Could you check a few things on this model? Use its own coordinates, in mm. Face numbers are marked on the shaded views. A direction names the side the tool comes from. Round coordinates to 2 decimals unless told otherwise and drop trailing zeros. Write each loop counter-clockwise with the first axis right and the second up, starting at its lowest first coordinate (ties: lowest second). Pieces come first, ordered by that corner, then holes. Notation, with made-up numbers: (13, 84.5) -> (25, 84.5) arc R12 ccw to (25, 96.5) -> close; hole circle Ø4 at (83.25, 45). An arc over 180 degrees is marked (long way). Answer in a Markdown table with one row per item.
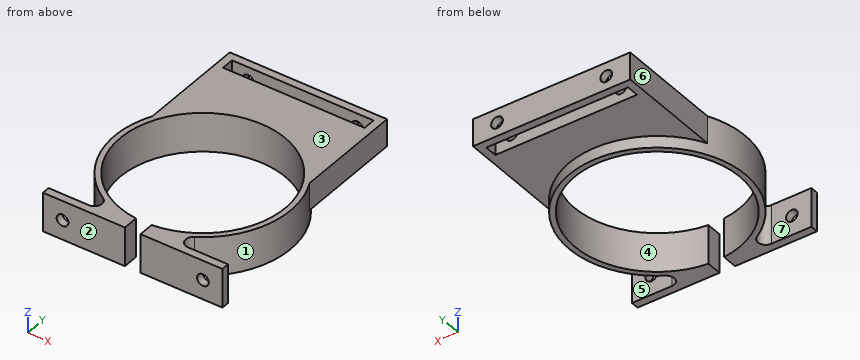
Autodesk Inventor part; units mm, degrees
ref_plane "YZ Plane" through (0, 0, 0) normal (1, 0, 0) x (0, 1, 0)
ref_plane "XZ Plane" through (0, 0, 0) normal (0, 1, 0) x (-1, 0, 0)
ref_plane "XY Plane" through (0, 0, 0) normal (0, 0, 1) x (1, 0, 0)
sketch "Sketch1" plane through (0, 0, 0) normal (0, 0, 1) x (1, 0, 0)
  circle A0 centre (0, 0) radius 21.15 construction
  line L0 (-18, -25) -> (18, -25) construction
  line L1 (-18, -25) -> (-18, -38.1522) construction
  line L2 (18, -25) -> (18, -38.1522) construction
  line L3 (-23, -23) -> (-23, -25)
  line L4 (-23, -25) -> (-2, -25)
  line L5 (-2, -21.0552) -> (-2, -25)
  line L6 (2, -21.0552) -> (2, -25)
  line L7 (2, -25) -> (23, -25)
  line L8 (23, -25) -> (23, -23)
  line L9 (23, -23) -> (12.7162, -23)
  line L10 (-23, -23) -> (-12.7162, -23)
  arc A1 (11.6803, -19.2892) -> (-11.6803, -19.2892) centre (0, 0) ccw
  arc A2 (2, -21.0552) -> (-2, -21.0552) centre (0, 0) ccw
  arc A3 (11.6803, -19.2892) -> (12.7162, -23) centre (12.7162, -21) ccw
  arc A4 (-12.7162, -23) -> (-11.6803, -19.2892) centre (-12.7162, -21) ccw
  point P0 (0, -25)
  dimension "d13" = 42.3
  dimension "d1" = 25
  dimension "d2" = 36
  dimension "d3" = 2
  dimension "d4" = 1.4
  dimension "d5" = 5
  dimension "d6" = 2
  dimension "d7" = 4
extrude "Extrusion1" add sketch "Sketch1" along normal blind 10
sketch "Sketch2" plane through (2, -25, 0) normal (0, -1, 0) x (1, 0, 0)
  circle A0 centre (16, 5) radius 1.5
  line L0 (21, 0) -> (21, 10)
  point P0 (-2, 0)
  point P1 (16, 0)
  point P2 (16, 0)
  point P3 (16, 0)
  point P4 (21, 5)
  dimension "d10" = 3
extrude "Extrusion2" cut sketch "Sketch2" against normal up to surface (2 mm away)
mirror "Mirror1" about plane through (0, 0, 0) normal (1, 0, 0) of "Extrusion2"
sketch "Sketch3" plane through (0, 0, 10) normal (0, 0, 1) x (1, 0, 0)
  arc A0 (21.9303, 5.25) -> (-21.9303, 5.25) centre (0, 0) ccw
  line L0 (-18.15, 35.75) -> (18.15, 35.75)
  line L1 (18.15, 35.75) -> (18.15, 32.55)
  line L2 (18.15, 32.55) -> (-18.15, 32.55)
  line L3 (-18.15, 32.55) -> (-18.15, 35.75)
  line L4 (-20.15, 37.75) -> (20.15, 37.75)
  line L5 (20.15, 37.75) -> (20.15, 10.1232)
  arc A1 (11.6803, -19.2892) -> (-11.6803, -19.2892) centre (0, 0) ccw
  line L6 (-20.15, 37.75) -> (-20.15, 10.1232)
  point P0 (0, 35.75)
  dimension "d14" = 3.2
  dimension "d15" = 36.3
  dimension "d16" = 10
  dimension "d17" = 2
  dimension "d18" = 2
  dimension "d19" = 2
extrude "Extrusion3" add sketch "Sketch3" against normal blind 7
sketch "Sketch4" plane through (-20.15, 37.75, 10) normal (0, 1, 0) x (1, 0, 0)
  circle A0 centre (34.15, 3.5) radius 1.5
  circle A1 centre (6.15, 3.5) radius 1.5
  line L0 (34.15, 3.5) -> (6.15, 3.5) construction
  line L1 (0, 7) -> (40.3, 7) construction
  line L2 (0, 0) -> (0, 7)
  point P0 (20.15, 10)
  point P1 (20.15, 3.5)
  point P2 (20.15, 7)
  point P3 (0, 3.5)
  dimension "d22" = 3
  dimension "d23" = 3
  dimension "d24" = 28
extrude "Extrusion4" cut sketch "Sketch4" against normal blind 12
properties part number "OmegaRing" material "ABS Plastic"
1) For the marked faces 5, 6 and 7, which set-ups out of +Z, -Z, +X, -X, +Y, -Y let a thin tool reach every point of the face, with its end or its side?
Findings:
| item | result |
|---|---|
| face 5 | +Z, -Z, +X |
| face 6 | +Z, -Z, -X, +Y |
| face 7 | +Z, -Z, -X |
2) Please list where these lines run through material, in increasing order: line 1 (X direction, y = 30.5, z = 6.5); line 2 (Z direction, x = -18, y = -23.7); line 3 (Z direction, x = -14, y = 37.1).
Findings:
| item | result |
|---|---|
| line 1 | x = -20.15 to -15.5, -12.5 to 12.5, 15.5 to 20.15 |
| line 2 | z = 0 to 3.5, 6.5 to 10 |
| line 3 | z = 3 to 5, 8 to 10 |
3) Imagine slicing it at C-C, the plane x = 0. Please give me the cut outline in (y, z), plus the area to 3 significant figures.
Findings:
| item | result |
|---|---|
| outline | (21.15, 0) -> (22.55, 0) -> (22.55, 3) -> (32.55, 3) -> (32.55, 10) -> (21.15, 10) -> close; (35.75, 3) -> (37.75, 3) -> (37.75, 10) -> (35.75, 10) -> close |
| area | 98.0 mm^2 |
4) Imagine slicing it at A-A, the plane y = 0. Please give me the cut outline in (x, z).
Findings:
| item | result |
|---|---|
| outline | (-22.55, 0) -> (-21.15, 0) -> (-21.15, 10) -> (-22.55, 10) -> close; (21.15, 0) -> (22.55, 0) -> (22.55, 10) -> (21.15, 10) -> close |
5) For pin 1 (1 mm diameter, centred on y = 34.5, z = 5.5, fed in from +X); pin 2 (1 mm diameter, centred on y = 34.5, z = 8, fed in from -X); pin 3 (2.5 mm diameter, centred on x = -14, z = 6.5, fed in from +Y), each with a flat end and sliding along its axis, tell me the tip position at first contact or that it passes through.
Findings:
| item | result |
|---|---|
| pin 1 | stops at x = 20.15 |
| pin 2 | stops at x = -20.15 |
| pin 3 | stops at y = 25.75 |
6) Thinking about a two-plate mould opening in Y: for the marked faces 1, 2, 3 and 4, which applies, +Y half, -Y half, draft (parallel to the pull), parting line (faces both ways), or undercut?
Findings:
| item | result |
|---|---|
| face 1 | undercut |
| face 2 | -Y half |
| face 3 | draft |
| face 4 | undercut |
7) Imagine slicing it at D-D, the plane y = 27.5. Please give me the cut outline in (x, z), plus the area to 3 significant figures.
Findings:
| item | result |
|---|---|
| outline | (-20.15, 3) -> (20.15, 3) -> (20.15, 10) -> (-20.15, 10) -> close; hole circle Ø3 at (-14, 6.5); hole circle Ø3 at (14, 6.5) |
| area | 268 mm^2 |
8) Imagine slicing it at B-B, the plane x = -6. Please give me the cut outline in (y, z).
Findings:
| item | result |
|---|---|
| outline | (-25, 0) -> (-20.28, 0) -> (-20.28, 10) -> (-25, 10) -> close; (20.28, 0) -> (21.74, 0) -> (21.74, 3) -> (32.55, 3) -> (32.55, 10) -> (20.28, 10) -> close; (35.75, 3) -> (37.75, 3) -> (37.75, 10) -> (35.75, 10) -> close |
